For this review, use the dimensioned drawing (mm, ordinates from the lowest corner) and the shaded views. Give positions to 0.01 mm unless a question says otherwise; leave off trailing zeros. Write each loop counter-clockwise with the first axis right and the second up, starting at its lowest first coordinate (ties: lowest second). Pieces come first, ordered by that corner, then holes.
1) We need section C-C on x = 56. Give the boundary of the cut face in (y, z).
2) Wall thickness on line 1 along Y through (x, z) = (6, 0.65); line 2 along X through (y, z) = (18.5, 0.85) (1 decimal); line 3 along X through (y, z) = (5, 1.9): over which ranges is each line inside the solid? List them lowest first.
3) For P1, Ø1.8, axis at x = 6, y = 4.75, coming from the +Z side; P2, Ø0.9, axis at y = 18, z = 1, coming from the +X side, all flat-tipped, find the tip position at first contact; note any pin that passes through.
4) We need section D-D on z = 1.95. Give the number of separate pieces and of enclosed holes in the cut face, and give its area (3 significant figures).
5) We need section B-B on y = 30.25. Give the boundary of the cut face in (x, z), and give its area (3 significant figures).
6) We need section A-A on x = 46. Give the boundary of the cut face in (y, z) (1 decimal).
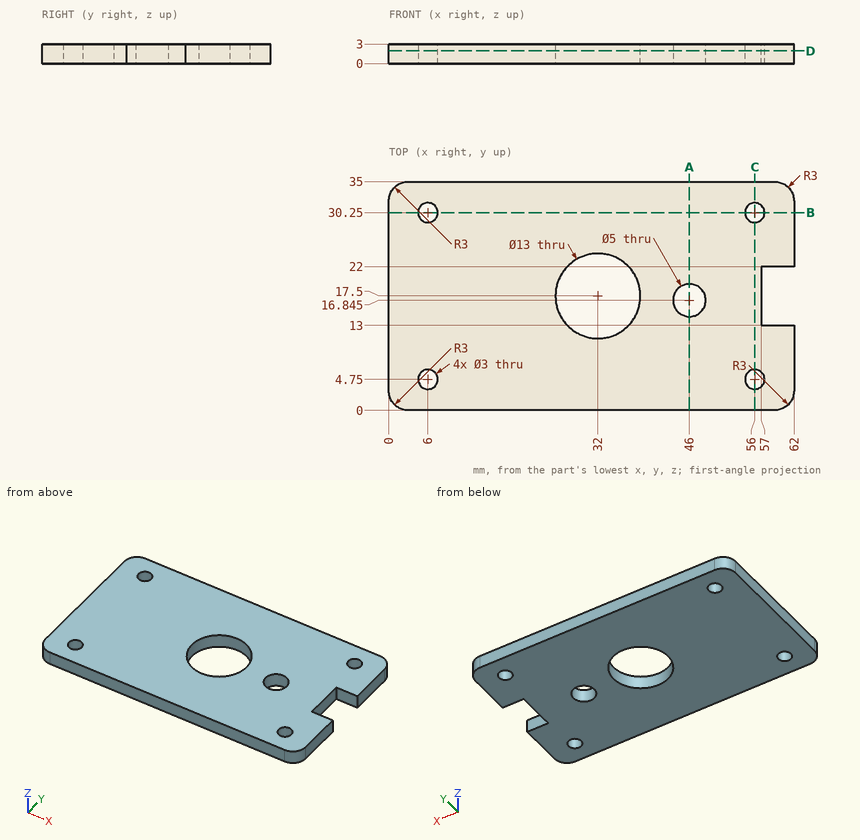
Results list:
1. outline: (0, 0) - (3.25, 0) - (3.25, 3) - (0, 3) - close; (6.25, 0) - (28.75, 0) - (28.75, 3) - (6.25, 3) - close; (31.75, 0) - (35, 0) - (35, 3) - (31.75, 3) - close
2. line 1: y = 0 to 3.25, 6.25 to 28.75, 31.75 to 35
2. line 2: x = 0 to 25.6, 38.4 to 44.1, 47.9 to 57
2. line 3: x = 0 to 4.52, 7.48 to 54.52, 57.48 to 62
3. P1: passes through
3. P2: stops at x = 57
4. separate pieces: 1
4. enclosed holes: 6
4. area: 1,940 mm2
5. outline: (0, 0) - (4.5, 0) - (4.5, 3) - (0, 3) - close; (7.5, 0) - (54.5, 0) - (54.5, 3) - (7.5, 3) - close; (57.5, 0) - (62, 0) - (62, 3) - (57.5, 3) - close
5. area: 168 mm2
6. outline: (0, 0) - (14.3, 0) - (14.3, 3) - (0, 3) - close; (19.3, 0) - (35, 0) - (35, 3) - (19.3, 3) - close
